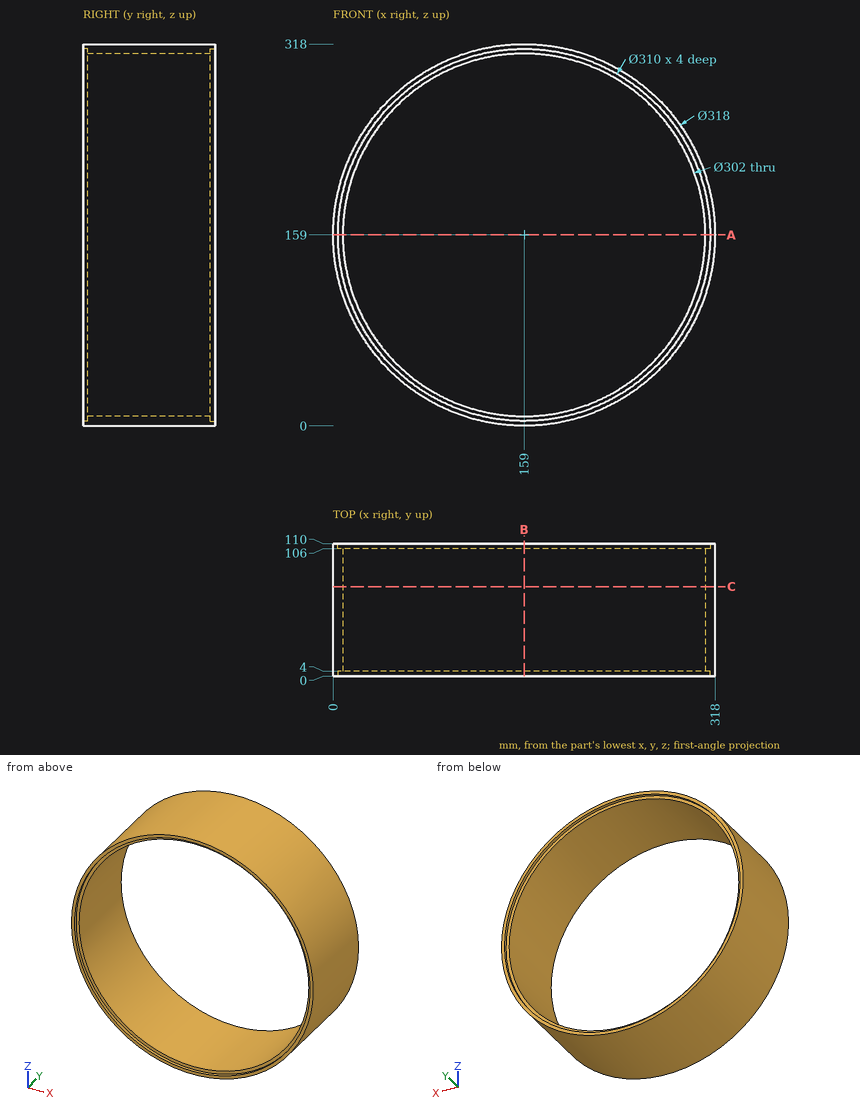
Can you work these out from the drawing? Everything is in mm from the part's minimum corner. Give positions to 0.01 mm unless a question says otherwise; leave off trailing zeros. Loops run counter-clockwise (first coordinate to the right, second up) from the corner with the lowest first, then second, coordinate; pieces in that order, holes last. Notation, with made-up numbers: (20.25, -27) - (43.25, -27) arc R8 cw to (43.25, -16) - close; hole circle Ø2 at (81.25, -5). An arc over 180 degrees is marked (long way). Answer as a JSON object with one key per item and string values.
Q1. Imagine slicing it at A-A on z = 159. Write out the boundary of the cut face in (x, y).
Geometry says:
{"outline": "(0, 0) - (4, 0) - (4, 4) - (8, 4) - (8, 106) - (4, 106) - (4, 110) - (0, 110) - close; (310, 4) - (314, 4) - (314, 0) - (318, 0) - (318, 110) - (314, 110) - (314, 106) - (310, 106) - close"}
Q2. Imagine slicing it at C-C on y = 74.5. Write out the boundary of the cut face in (x, z), plus the area to 3 significant figures.
Geometry says:
{"outline": "circle Ø318 at (159, 159); hole circle Ø302 at (159, 159)", "area": "7,790 mm²"}
Q3. Will these pins go through, and if not, where does the flat tip stop? P1, Ø1, axis at y = 42.5, z = 158, coming from the -X side; P2, Ø8, axis at x = 119.5, y = 18.5, coming from the -Z side; P3, Ø12, axis at y = 42, z = 206, coming from the -X side.
Geometry says:
{"P1": "x = 0", "P2": "z = 4.01", "P3": "x = 5.38"}
Q4. Imagine slicing it at B-B on x = 159. Write out the boundary of the cut face in (y, z), plus the area to 3 significant figures.
Geometry says:
{"outline": "(0, 0) - (110, 0) - (110, 4) - (106, 4) - (106, 8) - (4, 8) - (4, 4) - (0, 4) - close; (0, 314) - (4, 314) - (4, 310) - (106, 310) - (106, 314) - (110, 314) - (110, 318) - (0, 318) - close", "area": "1,700 mm²"}
Q5. If I drill on L1, parallel to X at y = 1.1, z = 159; L2, parallel to Z at x = 159, y = 42; L3, parallel to X at y = 87.5, z = 156.5, over which ranges is the centre line in solid material (lowest first)?
Geometry says:
{"L1": "0 to 4, 314 to 318", "L2": "0 to 8, 310 to 318", "L3": "0.02 to 8.02, 309.98 to 317.98"}
